Here's how the part is built. I have some questions about the finished solid (model axes, mm). A direction names the side the tool comes from. Round coordinates to 2 decimals unless told otherwise and drop trailing zeros. Write each loop counter-clockwise with the first axis right and the second up, starting at its lowest first coordinate (ties: lowest second). Pieces come first, ordered by that corner, then holes. Notation, with made-up numbers: (63.25, 20) -> (80.25, 20) arc R26 ccw to (80.25, 48) -> close; hole circle Ø8 at (76.5, -22). An arc over 180 degrees is marked (long way). Put each result on its own line as item: value. Start each with the question number.
1. Suppose I cut it at B-B (x = 12). Please give me the cut outline in (y, z), then the cut area to 3 significant figures.
2. For pin 1 (3.5 mm diameter, centred on x = 17.61, z = -30, fed in from +Y); pin 2 (1.5 mm diameter, centred on y = 3, z = 2.5, fed in from -X); pin 3 (1.5 mm diameter, centred on x = 27, y = 3.5, fed in from -Z); pin 4 (1.5 mm diameter, centred on x = 4.5, y = 2, fed in from +Z), each with a flat end and sliding along its axis, tell me the tip position at first contact or that it passes through.
3. We'd pull the mould along Z, two halves only. Please class faces 5 (the face through (30, 2, -20)), 6 (the face through (5, 2, 0)), 7 (the face through (17.68, 2.46, -31.5)): +Z half, -Z half, draft (parallel to the pull), parting line (faces both ways), or undercut.
4. Suppose I cut it at D-D (x = 23.5). Please give me the cut outline in (y, z).
5. I need wall thicknesses on probe 1 along X at (y, z) = (3.4, -30); probe 2 along Z at (x, y) = (11, 2.1); probe 3 along Z at (x, y) = (21, 3.2). Which ranges of each line are inside material? Lowest first, please. Write a range as from..to.
6. Suppose I cut it at C-C (y = 3.7). Please give me the cut outline in (x, z).
7. Which directions (+Z, -Z, +X, -X, +Y, -Y) give clear straight access to the entire face, cutting with the end or side of a thin tool? Please do faces 1 (the face through (10, 2, 3)), 2 (the face through (20, 2, -43)), 3 (the face through (20, 2, 2)), 4 (the face through (10, 2, -42)).
8. Suppose I cut it at A-A (z = -30). Please give me the cut outline in (x, y), then the cut area to 3 significant figures.
```python
from build123d import *

# Parameters (mm, degrees)
SKETCH_1_R      = 1.5
EXTRUDE_1_DEPTH = 5


with BuildPart() as part:
    # 草图1 → 凸台-拉伸1 (new body)
    with BuildSketch(Plane(origin=(0, 0, 0), x_dir=(1, 0, 0), z_dir=(0, 1, 0))):
        Polygon((20, 40), (30, 40), (30, 0), (20, 0), (20, -5), (10, -5), (10, 0), (0, 0), (0, 40), (10, 40), (10, 45), (20, 45), align=None)
        with Locations(Location((12, 30, 0), (0, 0, 270))):
            Circle(SKETCH_1_R, mode=Mode.SUBTRACT)
        with Locations(Location((17.61050347, 30, 0), (0, 0, 270))):
            Circle(SKETCH_1_R, mode=Mode.SUBTRACT)
        with Locations(Location((18, 10, 0), (0, 0, 270))):
            Circle(SKETCH_1_R, mode=Mode.SUBTRACT)
        with Locations(Location((12, 10, 0), (0, 0, 270))):
            Circle(SKETCH_1_R, mode=Mode.SUBTRACT)
    extrude(amount=EXTRUDE_1_DEPTH)


solid = part.part
```
Verdict:
1. outline: (0, -45) -> (5, -45) -> (5, -31.5) -> (0, -31.5) -> close; (0, -28.5) -> (5, -28.5) -> (5, -11.5) -> (0, -11.5) -> close; (0, -8.5) -> (5, -8.5) -> (5, 5) -> (0, 5) -> close
1. area: 220 mm^2
2. pin 1: stops at y = 5
2. pin 2: stops at x = 10
2. pin 3: stops at z = -40
2. pin 4: stops at z = 0
3. face 5: draft
3. face 6: +Z half
3. face 7: undercut
4. outline: (0, -40) -> (5, -40) -> (5, 0) -> (0, 0) -> close
5. probe 1: x = 0..10.5, 13.5..16.11, 19.11..30
5. probe 2: z = -45..-31.12, -28.88..-11.12, -8.88..5
5. probe 3: z = -40..0
6. outline: (0, -40) -> (10, -40) -> (10, -45) -> (20, -45) -> (20, -40) -> (30, -40) -> (30, 0) -> (20, 0) -> (20, 5) -> (10, 5) -> (10, 0) -> (0, 0) -> close; hole circle Ø3 at (12, -30); hole circle Ø3 at (12, -10); hole circle Ø3 at (17.61, -30); hole circle Ø3 at (18, -10)
7. face 1: +Z, -X, +Y, -Y
7. face 2: -Z, +X, +Y, -Y
7. face 3: +Z, +X, +Y, -Y
7. face 4: -Z, -X, +Y, -Y
8. outline: (0, 0) -> (10.5, 0) -> (10.5, 5) -> (0, 5) -> close; (13.5, 0) -> (16.11, 0) -> (16.11, 5) -> (13.5, 5) -> close; (19.11, 0) -> (30, 0) -> (30, 5) -> (19.11, 5) -> close
8. area: 120 mm^2
